Read the model definition and answer for the solid it produces. Units are mm, in the model's axes. Coordinates: 2 decimals unless noted, no trailing zeros. Write each loop counter-clockwise with the first axis right and the second up, starting at its lowest first coordinate (ties: lowest second). Pieces come first, ordered by that corner, then holes.
(1) The part is cut by section A-A, the plane z = 1.3. Determine the outline of the cut face in (x, y).
(2) Straight lines are drawn through the part: line 1 along X through (y, z) = (35, 0.95); line 2 along Y through (x, z) = (-30, 2.6); line 3 along X through (y, z) = (-24.5, 0.3). For each, find the intervals that lie inside material, in ascending order.
(3) Determine the mould class of faces 1 (the flat face through (0, -25, 1)), 2 (the flat face through (0, 12, 3)), 3 (the cylindrical face through (-32.468, -27.213, 1.479)) for opening direction Y: pulls with the +Y half, pulls with the -Y half, needs draft (parallel to the pull), parting line crosses it, or undercut.
(4) The part is cut by section C-C, the plane x = -1. Determine the outline of the cut face in (y, z).
(5) The part is cut by section B-B, the plane y = -17.5. Determine the outline of the cut face in (x, z), and give its area (3 significant figures).
(6) Given pin 1 (1 mm diameter, centred on y = 12, z = 1.5, fed in from +X); pin 2 (1.5 mm diameter, centred on y = 27, z = 2, fed in from +X), each flat-ended and moving along its own axis, determine where each tip first touches the part or whether it passes through.
(7) The part is cut by section D-D, the plane x = -37.5. Determine the outline of the cut face in (y, z).
```python
from build123d import *

# Parameters (mm, degrees)
F0_R     = 9.95
F1_DEPTH = 3


with BuildPart() as f1:
    # F0 (on Top) → F1 (new body)
    with BuildSketch(Plane.XY):
        with BuildLine():
            Line((-11.18034, 25), (-14.433757, 25))
            Line((-14.433757, 25), (-21.650635, 12.5))
            Line((-21.650635, 12.5), (-28.867513, 0))
            Line((-28.867513, 0), (-27.240805, -2.817542))
            ThreePointArc((-27.240805, -2.817542), (-43.30127, -25), (-16.060465, -22.182458))
            Line((-16.060465, -22.182458), (-14.433757, -25))
            Line((-14.433757, -25), (0, -25))
            Line((0, -25), (14.433757, -25))
            Line((14.433757, -25), (16.060465, -22.182458))
            ThreePointArc((16.060465, -22.182458), (43.30127, -25), (27.240805, -2.817542))
            Line((27.240805, -2.817542), (28.867513, 0))
            Line((28.867513, 0), (21.650635, 12.5))
            Line((21.650635, 12.5), (14.433757, 25))
            Line((14.433757, 25), (11.18034, 25))
            ThreePointArc((11.18034, 25), (0, 50), (-11.18034, 25))
        make_face()
        with Locations((-30.310889, -17.5)):
            Circle(F0_R, mode=Mode.SUBTRACT)
        with Locations((30.310889, -17.5)):
            Circle(F0_R, mode=Mode.SUBTRACT)
        with BuildLine():
            ThreePointArc((-9.526279, 5.5), (0, 11), (9.526279, 5.5))
            ThreePointArc((9.526279, 5.5), (9.526279, -5.5), (0, -11))
            ThreePointArc((0, -11), (-9.526279, -5.5), (-9.526279, 5.5))
        make_face(mode=Mode.SUBTRACT)
        with BuildLine():
            ThreePointArc((0, 25.05), (-7.035712, 42.035712), (9.95, 35))
            ThreePointArc((9.95, 35), (7.035712, 27.964288), (0, 25.05))
        make_face(mode=Mode.SUBTRACT)
    extrude(amount=F1_DEPTH)


solid = f1.part
```
Computed:
1. outline: (-28.87, 0) - (-27.24, -2.82) arc R15 ccw (long way) to (-16.06, -22.18) - (-14.43, -25) - (14.43, -25) - (16.06, -22.18) arc R15 ccw (long way) to (27.24, -2.82) - (28.87, 0) - (14.43, 25) - (11.18, 25) arc R15 ccw (long way) to (-11.18, 25) - (-14.43, 25) - close; hole circle Ø19.9 at (-30.31, -17.5); hole circle Ø22 at (0, 0); hole (0, 25.05) arc R9.95 ccw to (9.95, 35) arc R9.95 ccw (long way) to start; hole circle Ø19.9 at (30.31, -17.5)
2. line 1: x = -15 to -9.95, 9.95 to 15
2. line 2: y = -32.5 to -27.45, -7.55 to -2.5
2. line 3: x = -43.58 to -37.38, -23.24 to -17.04, -14.72 to 14.72, 17.04 to 23.24, 37.38 to 43.58
3. face 1: pulls with the -Y half
3. face 2: needs draft
3. face 3: undercut
4. outline: (-25, 0) - (-10.95, 0) - (-10.95, 3) - (-25, 3) - close; (10.95, 0) - (25.1, 0) - (25.1, 3) - (10.95, 3) - close; (44.9, 0) - (49.97, 0) - (49.97, 3) - (44.9, 3) - close
5. outline: (-45.31, 0) - (-40.26, 0) - (-40.26, 3) - (-45.31, 3) - close; (-20.36, 0) - (20.36, 0) - (20.36, 3) - (-20.36, 3) - close; (40.26, 0) - (45.31, 0) - (45.31, 3) - (40.26, 3) - close
5. area: 152 mm2
6. pin 1: stops at x = 22.23
6. pin 2: stops at x = 13.13
7. outline: (-30.66, 0) - (-24.38, 0) - (-24.38, 3) - (-30.66, 3) - close; (-10.62, 0) - (-4.34, 0) - (-4.34, 3) - (-10.62, 3) - close
